Part model, mm, in its own coordinate system. Coordinates: 2 decimals unless noted, no trailing zeros. Loops run counter-clockwise (first coordinate to the right, second up) from the corner with the lowest first, then second, coordinate; pieces in that order, holes last. Notation, with made-up numbers: M 53.25,18 L 111.25,18 A15 cw 111.25,47 Z; hole C 54,71.5 d6. An arc over 180 degrees is marked long. Use a Markdown table: item, result. Add a question column.
1) Wall check: probe 1 along X at (y, z) = (2.3, -23.5); probe 2 along X at (y, z) = (1, -24). Give the ranges that are in metal, low to high. Write a range as from..to.
2) Band-saw the part on A-A (y = 4). List the corners of the cut face in (x, z).
3) Band-saw the part on B-B (z = -17). List the corners of the cut face in (x, y).
4) Pin check, flat tip, straight feed: pin 1 Ø2 at (y, z) = (4, -31.5) entering from -X. Stop position of the tip, or through.
from build123d import *

# Parameters (mm, degrees)
SKETCH2_W           = 100
SKETCH2_H           = 55
BOSS_EXTRUDE1_DEPTH = 5
CUT_EXTRUDE2_REACH  = 116.237
CUT_EXTRUDE3_DEPTH  = 66


with BuildPart() as part:
    # Sketch2 → Boss-Extrude1 (new body)
    with BuildSketch(Plane(origin=(0, 0, 0), x_dir=(1, 0, 0), z_dir=(0, 1, 0))):
        with Locations((-50, 27.5)):
            Rectangle(SKETCH2_W, SKETCH2_H)
    extrude(amount=BOSS_EXTRUDE1_DEPTH)

    # Sketch5 → Cut-Extrude2 (cut, up to next)
    with BuildSketch(Plane.XY, mode=Mode.PRIVATE) as cut_extrude2_sk1:
        Polygon((0, 0), (-5, 5), (0, 5), align=None)
    cut_extrude2_tool1 = extrude(cut_extrude2_sk1.sketch, amount=-CUT_EXTRUDE2_REACH, mode=Mode.PRIVATE) & part.part
    add(cut_extrude2_tool1.solids().sort_by_distance((-1.666667, 3.333333, 0))[0], mode=Mode.SUBTRACT)

    # Sketch3 → Cut-Extrude3 (cut)
    with BuildSketch(Plane.XY):
        Polygon((-100, 0), (-95, 5), (-100, 5), align=None)
    extrude(amount=-CUT_EXTRUDE3_DEPTH, mode=Mode.SUBTRACT)


solid = part.part
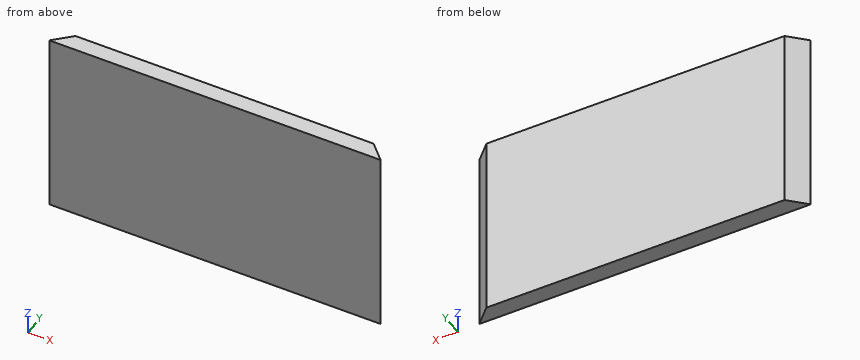
Entries:
| question | item | result |
|---|---|---|
| 1 | probe 1 | -97.7..-2.3 |
| 1 | probe 2 | -99..-1 |
| 2 | outline | M -96,-55 L -4,-55 L -4,0 L -96,0 Z |
| 3 | outline | M -100,0 L 0,0 L -5,5 L -95,5 Z |
| 4 | pin 1 | x = -97 |
